Build history of the part. All positions in model axes, mm. Face numbers are marked on the shaded views. Round coordinates to 2 decimals unless told otherwise and drop trailing zeros. Write each loop counter-clockwise with the first axis right and the second up, starting at its lowest first coordinate (ties: lowest second). Pieces come first, ordered by that corner, then holes. Notation, with made-up numbers: (47, 68.5) -> (65, 68.5) arc R33 ccw to (65, 98.5) -> close; hole circle Ø5 at (40, 35.5). An arc over 180 degrees is marked (long way). Answer in a Markdown table with one row per item. Add a question column.
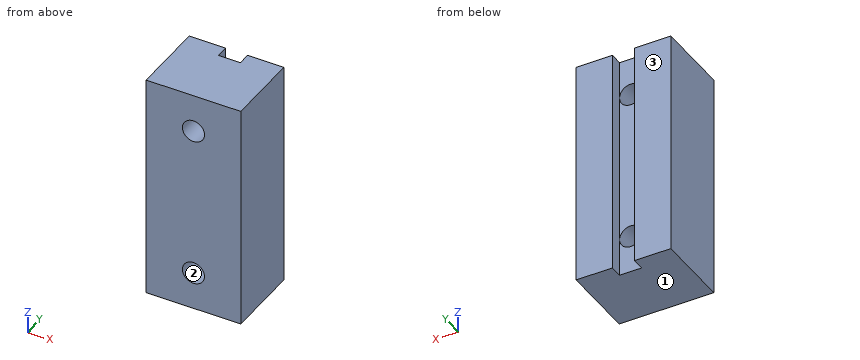
from build123d import *

# Parameters (mm, degrees)
SKETCH1_W           = 15
SKETCH1_H           = 36
BOSS_EXTRUDE1_DEPTH = 12
SKETCH2_R           = 1.75
CUT_EXTRUDE1_DEPTH  = 12
SKETCH3_W           = 3.5
SKETCH3_H           = 36
CUT_EXTRUDE2_DEPTH  = 2


with BuildPart() as part:
    # Sketch1 → Boss-Extrude1 (new body)
    with BuildSketch(Plane(origin=(0, 0, 0), x_dir=(1, 0, 0), z_dir=(0, 1, 0))):
        with Locations((7.5, 18)):
            Rectangle(SKETCH1_W, SKETCH1_H)
    extrude(amount=BOSS_EXTRUDE1_DEPTH)

    # Sketch2 → Cut-Extrude1 (cut)
    with BuildSketch(Plane(origin=(0, 12, 0), x_dir=(1, 0, 0), z_dir=(0, 1, 0))):
        with Locations(Location((7.5, 30, 0), (0, 0, 270))):
            Circle(SKETCH2_R)
        with Locations(Location((7.5, 6, 0), (0, 0, 270))):
            Circle(SKETCH2_R)
    extrude(amount=-CUT_EXTRUDE1_DEPTH, mode=Mode.SUBTRACT)

    # Sketch3 → Cut-Extrude2 (cut)
    with BuildSketch(Plane(origin=(0, 12, 0), x_dir=(1, 0, 0), z_dir=(0, 1, 0))):
        with Locations((7.5, 18)):
            Rectangle(SKETCH3_W, SKETCH3_H)
    extrude(amount=-CUT_EXTRUDE2_DEPTH, mode=Mode.SUBTRACT)


solid = part.part
(1) Drop flat-ended pins along their axis: P1, Ø4.5, axis at x = 7.5, z = -30, coming from the -Y side; P2, Ø1.8, axis at x = 7, z = -34, coming from the +Y side. Give the stop position or say it passes through.
(2) Mould opens along Z. For the marked faces 1, 2 and 3 say: pulls with the +Z half, pulls with the -Z half, needs draft (parallel to the pull), parting line crosses it, or undercut.
(3) Saw through at A-A (x = 7.5). List the corners of the cut face in (y, z), plus the area to 3 significant figures.
(4) Saw through at B-B (y = 1). List the corners of the cut face in (x, z).
(5) Saw through at D-D (z = -19). List the corners of the cut face in (x, y), plus the area to 3 significant figures.
(6) Probe line 1 along Z through (x, y) = (7.5, 7.25); line 2 along X through (y, z) = (3, -6); line 3 along Z through (x, y) = (9, 1). List the from-to ranges inside material, lowest first.
(7) Saw through at C-C (z = -30.5). List the corners of the cut face in (x, y).
Answer sheet:
| question | item | result |
|---|---|---|
| 1 | P1 | stops at y = 0 |
| 1 | P2 | stops at y = 10 |
| 2 | face 1 | pulls with the -Z half |
| 2 | face 2 | undercut |
| 2 | face 3 | needs draft |
| 3 | outline | (0, -36) -> (10, -36) -> (10, -31.75) -> (0, -31.75) -> close; (0, -28.25) -> (10, -28.25) -> (10, -7.75) -> (0, -7.75) -> close; (0, -4.25) -> (10, -4.25) -> (10, 0) -> (0, 0) -> close |
| 3 | area | 290 mm² |
| 4 | outline | (0, -36) -> (15, -36) -> (15, 0) -> (0, 0) -> close; hole circle Ø3.5 at (7.5, -30); hole circle Ø3.5 at (7.5, -6) |
| 5 | outline | (0, 0) -> (15, 0) -> (15, 12) -> (9.25, 12) -> (9.25, 10) -> (5.75, 10) -> (5.75, 12) -> (0, 12) -> close |
| 5 | area | 173 mm² |
| 6 | line 1 | z = -36 to -31.75, -28.25 to -7.75, -4.25 to 0 |
| 6 | line 2 | x = 0 to 5.75, 9.25 to 15 |
| 6 | line 3 | z = -36 to -30.9, -29.1 to -6.9, -5.1 to 0 |
| 7 | outline | (0, 0) -> (5.82, 0) -> (5.82, 10) -> (5.75, 10) -> (5.75, 12) -> (0, 12) -> close; (9.18, 0) -> (15, 0) -> (15, 12) -> (9.25, 12) -> (9.25, 10) -> (9.18, 10) -> close |
